Build history of the part. All positions in model axes, mm. A direction names the side the tool comes from. Coordinates: 2 decimals unless noted, no trailing zeros. Loops run counter-clockwise (first coordinate to the right, second up) from the corner with the lowest first, then second, coordinate; pieces in that order, holes last. Notation, with made-up numbers: (20.25, 33.5) - (44.25, 33.5) arc R20 cw to (44.25, 47.5) - close; hole circle Ø10 at (87, 22.25). An arc over 180 degrees is marked (long way). One line per item, written item: value.
```python
from build123d import *

# Parameters (mm, degrees)
F1_DEPTH = 3
F0_W     = 12
F0_H     = 3
F0_W_2   = 3
F0_H_2   = 17
F2_DEPTH = 15
F3_R     = 1.75
F4_DEPTH = 25
F3_R_2   = 4.5
F3_R_3   = 3.5
F5_DEPTH = 1
F6_DEPTH = 1
F7_SIZE2 = 2.1
F7_SIZE  = 3.5
F8_R     = 1.6
F9_DEPTH = 25


with BuildPart() as f1:
    # F0 (on Top) → F1 (new body)
    with BuildSketch(Plane.XY):
        Polygon((-4.5, -10), (7.5, 7), (-4.5, 7), align=None)
    extrude(amount=F1_DEPTH)

    # F0 (on Top) → F2 (join)
    with BuildSketch(Plane.XY):
        with Locations((1.5, 8.5)):
            Rectangle(F0_W, F0_H)
        with Locations((-6, 8.5)):
            Rectangle(F0_W_2, F0_H)
        with Locations((-6, -1.5)):
            Rectangle(F0_W_2, F0_H_2)
    extrude(amount=F2_DEPTH)

    # F3 (on face) → F4 (cut)
    with BuildSketch(Plane.XZ.offset(-7)):
        with Locations((0.5, 9)):
            Circle(F3_R)
    extrude(amount=-F4_DEPTH, mode=Mode.SUBTRACT)

    # F3 (on face) → F5 (join)
    with BuildSketch(Plane.XZ.offset(-7)):
        with Locations((0.5, 9)):
            Circle(F3_R_2)
        with Locations((0.5, 9)):
            Circle(F3_R_3, mode=Mode.SUBTRACT)
    extrude(amount=F5_DEPTH)

    # F3 (on face) → F6 (join)
    with BuildSketch(Plane.XZ.offset(-7)):
        with Locations((0.5, 9)):
            Circle(F3_R_3)
        with Locations((0.5, 9)):
            Circle(F3_R, mode=Mode.SUBTRACT)
    extrude(amount=F6_DEPTH)

    # F7
    f7_edges = [f1.edges().sort_by_distance(p)[0] for p in [
        (-1.25, 6, 9),
    ]]
    chamfer(f7_edges, length=F7_SIZE, length2=F7_SIZE2)

    # F8 (on face) → F9 (cut)
    with BuildSketch(Plane(origin=(-7.5, 0, 0), x_dir=(0, -1, 0), z_dir=(-1, 0, 0))):
        with Locations((3.342046, 9.021713)):
            Circle(F8_R)
    extrude(amount=-F9_DEPTH, mode=Mode.SUBTRACT)


solid = f1.part
```
Item 1: Probe probe 1 along X at (y, z) = (9.85, 9); probe 2 along X at (y, z) = (5.5, 5.25); probe 3 along Y at (x, z) = (-3.5, 11). List the from-to ranges inside material, lowest first. Write a range as from..to.
Check result:
probe 1: x = -7.5..-1.25, 2.25..7.5
probe 2: x = -7.5..-4.5
probe 3: y = 6..10
Item 2: Cut at A-A, the plane z = 3.5. Write the cut outline in (x, y).
Check result:
outline: (-7.5, -10) - (-4.5, -10) - (-4.5, 7) - (7.5, 7) - (7.5, 10) - (-7.5, 10) - close
Item 3: Drop flat-ended pins along their axis: P1, Ø6, axis at x = 3, z = 11, coming from the -Y side; P2, Ø2.5, axis at x = 2, z = 7.5, coming from the -Y side; P3, Ø6, axis at x = 4.5, y = -3.5, coming from the -Z side. Give the stop position or say it passes through.
Check result:
P1: stops at y = 6
P2: stops at y = 6.8
P3: passes through
Item 4: Cut at B-B, the plane x = 5.5. Write the cut outline in (y, z), then the cut area to 3 significant figures.
Check result:
outline: (4.17, 0) - (10, 0) - (10, 15) - (7, 15) - (7, 3) - (4.17, 3) - close
area: 53.5 mm^2
Item 5: Pull direction X, two halves, no side cores. Call faces 1 (the face through (0.272, 9.746, 10.735)), 2 (the face through (1.416, -1.619, 1.479)), 3 (the face through (-5, 2, 15)), 4 (the face through (5.4, 7, 8.9)): released by +X, released by -X, zero draft, split by the parting line, or undercut.
Check result:
face 1: undercut
face 2: released by +X
face 3: zero draft
face 4: undercut
Item 6: Cut at C-C, the plane z = 9.5. Give the number of separate pieces and of enclosed holes in the cut face, then the cut area to 3 significant figures.
Check result:
separate pieces: 3
enclosed holes: 0
area: 74.8 mm^2
Item 7: Tool access for faces 5 (the face through (-2, 2, 0)), 6 (the face through (-0.09, 6.51, 13.46)): list every direction of +Z, -Z, +X, -X, +Y, -Y with a clear straight run to the whole face (end or side of a thin tool).
Check result:
face 5: -Z, +X, -X, +Y, -Y
face 6: -Y
